```python
from build123d import *

# Parameters (mm, degrees)
F1_DEPTH = 29
F2_W     = 36
F2_H     = 11
F3_DEPTH = 63.5
F5_DEPTH = 50


with BuildPart() as f1:
    # F0 (on Front) → F1 (new body, symmetric)
    with BuildSketch(Plane.XZ):
        with BuildLine():
            Line((-51.498091, 9), (-51.498091, 0))
            Line((-51.498091, 0), (53.501909, 0))
            Line((53.501909, 0), (53.501909, 9))
            Line((53.501909, 9), (64.501909, 9))
            ThreePointArc((64.501909, 9), (60.407201, 35.029386), (36.933812, 47))
            Line((36.933812, 47), (-34.929993, 47))
            ThreePointArc((-34.929993, 47), (-58.403383, 35.029386), (-62.498091, 9))
            Line((-62.498091, 9), (-51.498091, 9))
        make_face()
    extrude(amount=F1_DEPTH, both=True)

    # F2 (on Right) → F3 (cut, symmetric)
    with BuildSketch(Plane.YZ):
        with Locations((0, 41.5)):
            Rectangle(F2_W, F2_H)
    extrude(amount=F3_DEPTH, both=True, mode=Mode.SUBTRACT)

    # F4 (on Top) → F5 (cut, symmetric)
    with BuildSketch(Plane.XY):
        with BuildLine():
            Line((-18.498091, 4), (-37.498091, 4))
            ThreePointArc((-37.498091, 4), (-41.498091, 0), (-37.498091, -4))
            Line((-37.498091, -4), (-18.498091, -4))
            ThreePointArc((-18.498091, -4), (-14.498091, 0), (-18.498091, 4))
        make_face()
        with BuildLine():
            Line((20.501909, -4), (39.501909, -4))
            ThreePointArc((39.501909, -4), (43.501909, 0), (39.501909, 4))
            Line((39.501909, 4), (20.501909, 4))
            ThreePointArc((20.501909, 4), (16.501909, 0), (20.501909, -4))
        make_face()
    extrude(amount=F5_DEPTH, both=True, mode=Mode.SUBTRACT)


solid = f1.part
```
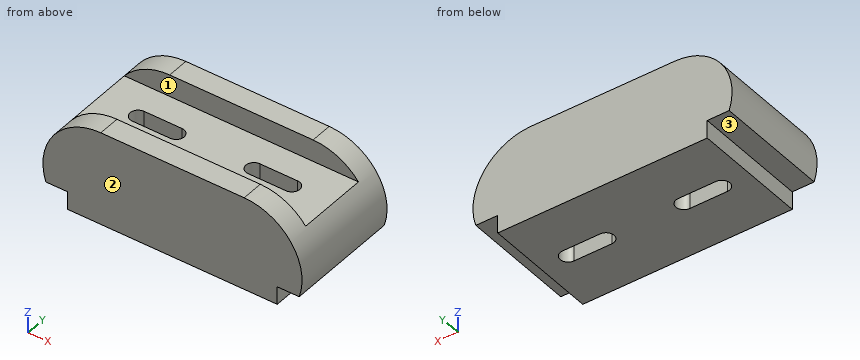
CAD build for the part. Positions are in the model's coordinates, mm. Face numbers are marked on the shaded views. A direction names the side the tool comes from. Round coordinates to 2 decimals unless told otherwise and drop trailing zeros. Loops run counter-clockwise (first coordinate to the right, second up) from the corner with the lowest first, then second, coordinate; pieces in that order, holes last. Notation, with made-up numbers: (58.5, 65.5) - (65.5, 65.5) arc R21 cw to (65.5, 95.5) - close; hole circle Ø10 at (85.5, 30). An arc over 180 degrees is marked (long way). Return JSON: item names as keys, results as strings. Group by question number.
Q1. Band-saw the part on A-A on x = 35.5. Give the cut face in (y, z).
Q2. Band-saw the part on B-B on y = 0. Give the cut face in (x, z).
Q3. Drill centre lines: line 1 along Y through (x, z) = (23.5, 12); line 2 along Y through (x, z) = (-35.5, 43.5); line 3 along X through (y, z) = (-3, 28). Where is each one in solid material? Low to high. Write a range as [from, to].
Q4. Band-saw the part on C-C on z = 40.5. Give the cut face in (x, y).
Q5. Band-saw the part on D-D on y = -15.5. Give the cut face in (x, z).
Q6. Tool access for the marked faces 1, 2 and 3: list every direction of +Z, -Z, +X, -X, +Y, -Y with a clear straight run to the whole face (end or side of a thin tool).
Q7. Flat gauge pins, fed straight in: pin 1 Ø4 at (y, z) = (-1.5, 20.5) entering from -X; pin 2 Ø12 at (y, z) = (5, 6) entering from +X; pin 3 Ø4.5 at (y, z) = (-11, 4) entering from -X. Where does each tip first touch, or does it go through?
Solutions:
{
 "1": {"outline": "(-29, 0) - (-4, 0) - (-4, 36) - (-18, 36) - (-18, 47) - (-29, 47) - close; (4, 0) - (29, 0) - (29, 47) - (18, 47) - (18, 36) - (4, 36) - close"},
 "2": {"outline": "(-62.5, 9) - (-51.5, 9) - (-51.5, 0) - (-41.5, 0) - (-41.5, 36) - (-57.67, 36) arc R29 ccw to start; (-14.5, 0) - (16.5, 0) - (16.5, 36) - (-14.5, 36) - close; (43.5, 0) - (53.5, 0) - (53.5, 9) - (64.5, 9) arc R29 ccw to (59.67, 36) - (43.5, 36) - close"},
 "3": {"line 1": "y = [-29, -4], [4, 29]", "line 2": "y = [-29, -18], [18, 29]", "line 3": "x = [-62.15, -40.14], [-15.85, 17.86], [42.15, 64.16]"},
 "4": {"outline": "(-53.23, -29) - (55.23, -29) - (55.23, -18) - (-53.23, -18) - close; (-53.23, 18) - (55.23, 18) - (55.23, 29) - (-53.23, 29) - close"},
 "5": {"outline": "(-62.5, 9) - (-51.5, 9) - (-51.5, 0) - (53.5, 0) - (53.5, 9) - (64.5, 9) arc R29 ccw to (59.67, 36) - (-57.67, 36) arc R29 ccw to start"},
 "6": {"face 1": "+Z, +X, -X", "face 2": "+Z, -Z, +X, -X, -Y", "face 3": "-Z, -X, +Y, -Y"},
 "7": {"pin 1": "stops at x = -63.93", "pin 2": "stops at x = 65.31", "pin 3": "stops at x = -51.5"}
}
